Job drawing, mm, ordinate dimensions from the low corner. One solid piece. A direction names the side the tool comes from. Give positions to 0.01 mm unless a question says otherwise; leave off trailing zeros. Loops run counter-clockwise (first coordinate to the right, second up) from the corner with the lowest first, then second, coordinate; pieces in that order, holes last. Notation, with made-up numbers: M 11,7 L 39,7 A16 ccw 39,25 Z; hole C 17,-30 d3. An arc over 180 degrees is marked long. Answer as CSV lines item,"result".
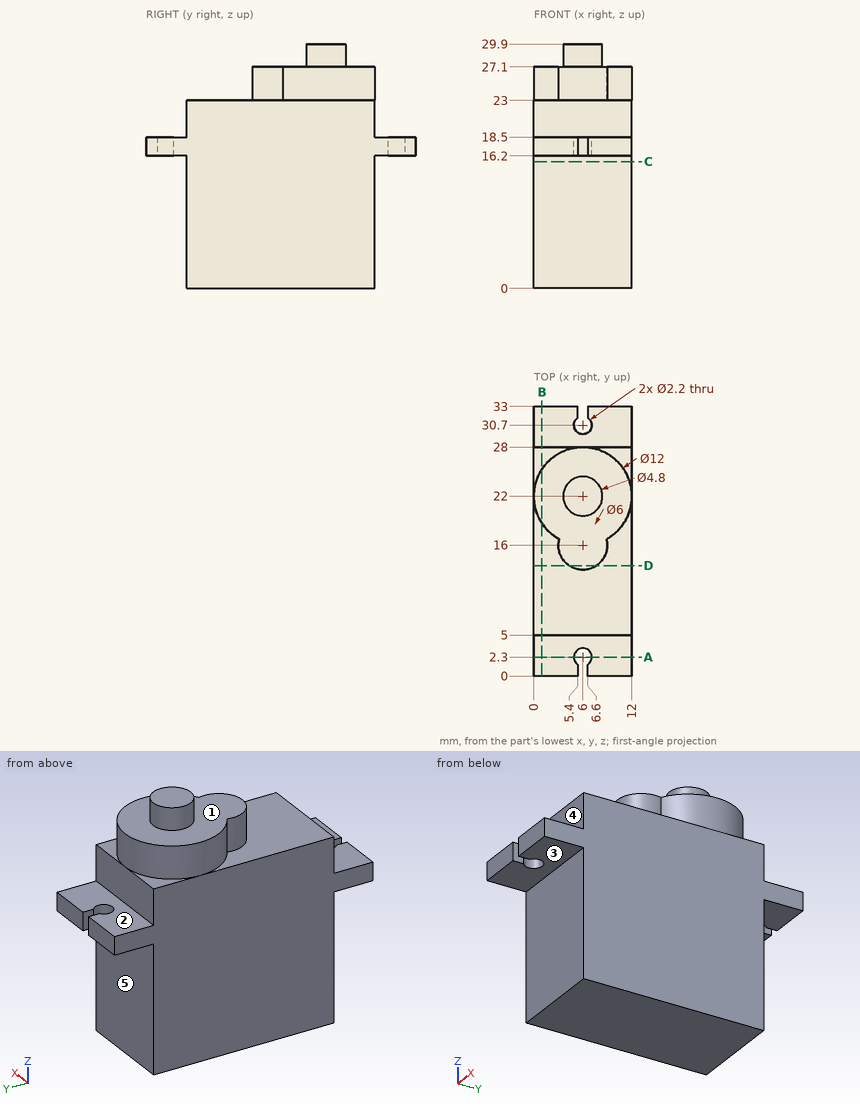
1) Band-saw the part on D-D on y = 13.5. Give the cut face in (x, z).
Answer below:
outline,"M 0,0 L 12,0 L 12,23 L 7.66,23 L 7.66,27.1 L 4.34,27.1 L 4.34,23 L 0,23 Z"
2) Band-saw the part on B-B on x = 1. Give the cut face in (y, z), and give its area (3 significant figures).
Answer below:
outline,"M 0,16.2 L 5,16.2 L 5,0 L 28,0 L 28,16.2 L 33,16.2 L 33,18.5 L 28,18.5 L 28,23 L 25.32,23 L 25.32,27.1 L 18.68,27.1 L 18.68,23 L 5,23 L 5,18.5 L 0,18.5 Z"
area,"579 mm^2"
3) Flat gauge pins, fed straight in: pin 1 (4 mm diameter, centred on x = 2.5, y = 9, fed in from +Z); pin 2 (1.5 mm diameter, centred on x = 3.5, y = 1.5, fed in from -Z); pin 3 (1.3 mm diameter, centred on x = 4, z = 21, fed in from +Y). Where does each tip first touch, or does it go through?
Answer below:
pin 1,"stops at z = 23"
pin 2,"stops at z = 16.2"
pin 3,"stops at y = 28"
4) Band-saw the part on A-A on y = 2.3. Give the cut face in (x, z).
Answer below:
outline,"M 0,16.2 L 4.9,16.2 L 4.9,18.5 L 0,18.5 Z; M 7.1,16.2 L 12,16.2 L 12,18.5 L 7.1,18.5 Z"
5) Which spindle directions (+Z, -Z, +X, -X, +Y, -Y) get a long thin tool onto all of the face, cutting with end or side? Do the marked faces 1, 2, 3, 4 and 5. Say none if no direction does.
Answer below:
face 1,"+Z"
face 2,"+Z, +X, -X, +Y"
face 3,"-Z, +X, -X, -Y"
face 4,"+Z, +X, -X, -Y"
face 5,"-Z, +X, -X, +Y"
6) Drill centre lines: line 1 (X direction, y = 30.7, z = 17); line 2 (Z direction, x = 4.25, y = 3.5); line 3 (Z direction, x = 1.75, y = 14.5). Where is each one in solid material? Low to high. Write a range as from..to.
Answer below:
line 1,"x = 0..4.9, 7.1..12"
line 2,"z = 16.2..18.5"
line 3,"z = 0..23"
7) Band-saw the part on C-C on z = 15.5. Give the cut face in (x, y).
Answer below:
outline,"M 0,5 L 12,5 L 12,28 L 0,28 Z"
